The figure shows three views and two pictorial views of one solid part (mm, origin at its lowest corner). Answer the questions. A direction names the side the tool comes from. Coordinates: 2 decimals unless noted, no trailing zeros. Loops run counter-clockwise (first coordinate to the right, second up) from the corner with the lowest first, then second, coordinate; pieces in that order, holes last. Notation, with made-up numbers: (-32.5, 41.25) -> (2.5, 41.25) arc R19 ccw to (2.5, 64.25) -> close; hole circle Ø4 at (20.25, -17.5). An arc over 180 degrees is marked (long way). Answer in a Markdown table with one row per item.
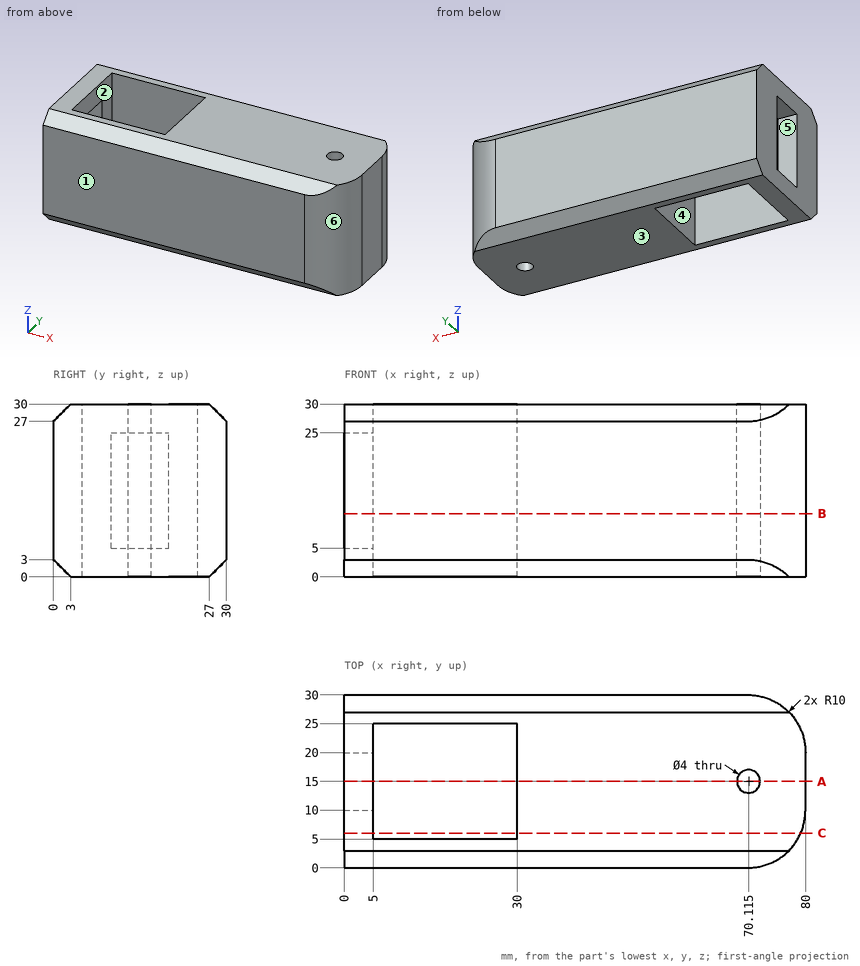
Item 1: A cutting plane is placed at B-B, the plane z = 11. Determine the outline of the cut face in (x, y) (3 decimals), plus the area to 3 significant figures.
Findings below:
| item | result |
|---|---|
| outline | (0, 0) -> (70, 0) arc R10 ccw to (80, 10) -> (80, 20) arc R10 ccw to (70, 30) -> (0, 30) -> (0, 20) -> (5, 20) -> (5, 25) -> (30, 25) -> (30, 5) -> (5, 5) -> (5, 10) -> (0, 10) -> close; hole circle Ø4 at (70.115, 15) |
| area | 1,790 mm2 |
Item 2: Determine the mould class of the marked faces 1, 2 and 3 for opening direction Y: +Y half, -Y half, draft (parallel to the pull), parting line (faces both ways), or undercut.
Findings below:
| item | result |
|---|---|
| face 1 | -Y half |
| face 2 | undercut |
| face 3 | draft |
Item 3: A cutting plane is placed at A-A, the plane y = 15. Determine the outline of the cut face in (x, z) (3 decimals), plus the area to 3 significant figures.
Findings below:
| item | result |
|---|---|
| outline | (0, 0) -> (5, 0) -> (5, 5) -> (0, 5) -> close; (0, 25) -> (5, 25) -> (5, 30) -> (0, 30) -> close; (30, 0) -> (68.115, 0) -> (68.115, 30) -> (30, 30) -> close; (72.115, 0) -> (80, 0) -> (80, 30) -> (72.115, 30) -> close |
| area | 1,430 mm2 |
Item 4: A cutting plane is placed at C-C, the plane y = 6. Determine the outline of the cut face in (x, z) (3 decimals), plus the area to 4 significant figures.
Findings below:
| item | result |
|---|---|
| outline | (0, 0) -> (5, 0) -> (5, 30) -> (0, 30) -> close; (30, 0) -> (79.165, 0) -> (79.165, 30) -> (30, 30) -> close |
| area | 1,625 mm2 |
Item 5: A tool of negligible diameter and unlimited length cuts with its end or side. For the marked faces 4, 5 and 6, from which of +Z, -Z, +X, -X, +Y, -Y can it reach the whole face along a straight path? Write none if from no direction.
Findings below:
| item | result |
|---|---|
| face 4 | +Z, -Z |
| face 5 | -X |
| face 6 | +Z, -Z, +X, -Y |
Item 6: Flat-ended cylindrical pins translate along their axes: pin 1 Ø3.5 at (x, y) = (70.11, 15) entering from -Z; pin 2 Ø4 at (x, y) = (21, 5) entering from -Z; pin 3 Ø2 at (y, z) = (6, 8.5) entering from +X; pin 4 Ø8 at (y, z) = (25, 18) entering from +X. Find the tip coordinate at first contact, or state that the pin passes through.
Findings below:
| item | result |
|---|---|
| pin 1 | passes through |
| pin 2 | stops at z = 0 |
| pin 3 | stops at x = 79.54 |
| pin 4 | stops at x = 79.95 |
Item 7: Find the intervals of material crossed by probe 1 along X at (y, z) = (14, 3.5); probe 2 along Y at (x, z) = (19.5, 11.5); probe 3 along X at (y, z) = (10.5, 8.5), in increasing order.
Findings below:
| item | result |
|---|---|
| probe 1 | x = 0 to 5, 30 to 68.38, 71.85 to 80 |
| probe 2 | y = 0 to 5, 25 to 30 |
| probe 3 | x = 30 to 80 |
